Check sheet for the drawn part. Datum: minimum x, y, z corner. Units: mm. A direction names the side the tool comes from. Round coordinates to 2 decimals unless told otherwise and drop trailing zeros. Loops run counter-clockwise (first coordinate to the right, second up) from the corner with the lowest first, then second, coordinate; pieces in that order, holes last.
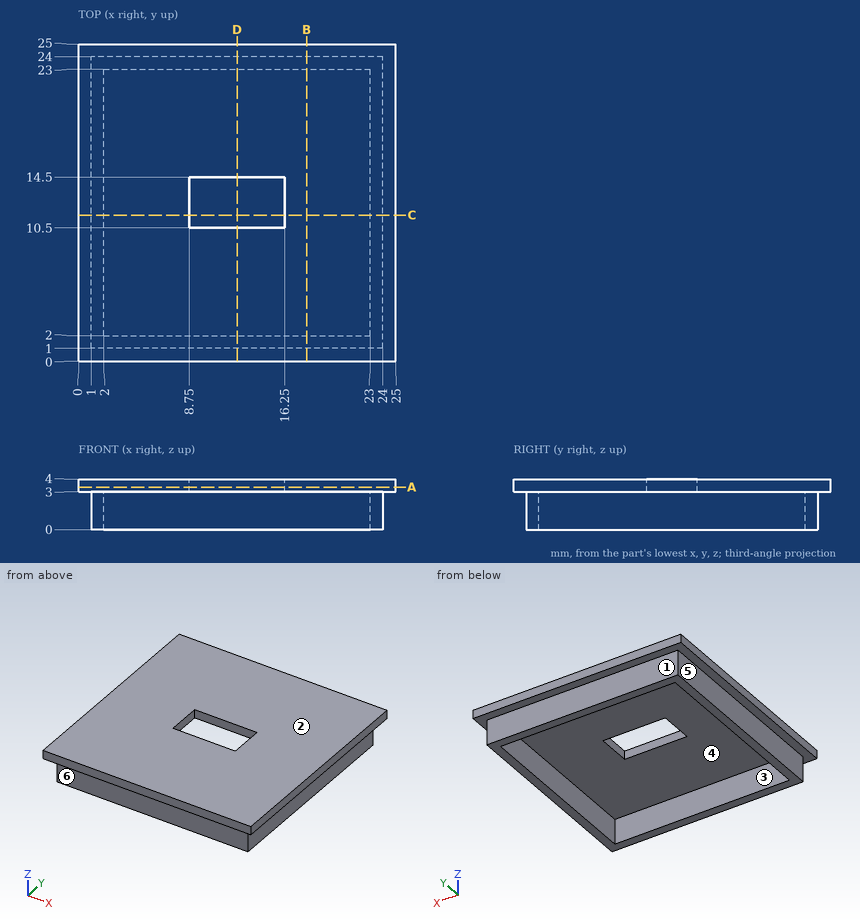
1) Scan lines: line 1 along Y through (x, z) = (17.5, 2.65); line 2 along Z through (x, y) = (15.75, 7.5). Record each from-to range of solid material in increasing order.
Report:
line 1: y = 1 to 2, 23 to 24
line 2: z = 3 to 4
2) Sectioned sample at D-D, the plane x = 12.5. Record the cut outline in (y, z).
Report:
outline: (0, 3) - (1, 3) - (1, 0) - (2, 0) - (2, 3) - (10.5, 3) - (10.5, 4) - (0, 4) - close; (14.5, 3) - (23, 3) - (23, 0) - (24, 0) - (24, 3) - (25, 3) - (25, 4) - (14.5, 4) - close
3) Sectioned sample at A-A, the plane z = 3.35. Record the cut outline in (x, y), then the cut area to 3 significant figures.
Report:
outline: (0, 0) - (25, 0) - (25, 25) - (0, 25) - close; hole (8.75, 10.5) - (16.25, 10.5) - (16.25, 14.5) - (8.75, 14.5) - close
area: 595 mm2
4) Gauge pin test, flat ends, axial feed: pin 1 (1.5 mm diameter, centred on x = 17, z = 2, fed in from -Y); pin 2 (0.5 mm diameter, centred on x = 13, z = 3.5, fed in from -Y); pin 3 (1.5 mm diameter, centred on y = 11.5, z = 1, fed in from +X); pin 4 (4 mm diameter, centred on x = 17, y = 12, fed in from -Z). Record the tip position at first contact, or that the pin passes through.
Report:
pin 1: stops at y = 1
pin 2: stops at y = 0
pin 3: stops at x = 24
pin 4: stops at z = 3
5) Mould release check, pull along Y, two halves, no side actions. Record for the marked faces 4, 5 and 6: +Y half, -Y half, draft (parallel to the pull), parting line (faces both ways), or undercut.
Report:
face 4: undercut
face 5: draft
face 6: -Y half
6) Sectioned sample at C-C, the plane y = 11.5. Record the cut outline in (x, z).
Report:
outline: (0, 3) - (1, 3) - (1, 0) - (2, 0) - (2, 3) - (8.75, 3) - (8.75, 4) - (0, 4) - close; (16.25, 3) - (23, 3) - (23, 0) - (24, 0) - (24, 3) - (25, 3) - (25, 4) - (16.25, 4) - close
7) Access from +Z, -Z, +X, -X, +Y, -Y to the whole of each face (thin tool, end or side, straight path). Record for the marked faces 1, 2 and 3.
Report:
face 1: -Z, +X, -X, +Y
face 2: +Z, +X, -X, +Y, -Y
face 3: -Z
8) Sectioned sample at B-B, the plane x = 18. Record the cut outline in (y, z).
Report:
outline: (0, 3) - (1, 3) - (1, 0) - (2, 0) - (2, 3) - (23, 3) - (23, 0) - (24, 0) - (24, 3) - (25, 3) - (25, 4) - (0, 4) - close
